```python
from build123d import *

# Parameters (mm, degrees)
SKETCH1_R                = 1.5
BOSS_EXTRUDE1_DEPTH      = 3.75
BOSS_EXTRUDE2_DEPTH      = 18
BOSS_EXTRUDE2_DEPTH_BACK = 7.5
CUT_EXTRUDE1_DEPTH       = 119.718371128
CUT_EXTRUDE1_DEPTH_BACK  = 3.5
SKETCH4_R                = 1.5
CHAMFER1_SIZE            = 2


with BuildPart() as part:
    # Sketch1 → Boss-Extrude1 (new, symmetric)
    with BuildSketch(Plane(origin=(0, 0, 0), x_dir=(1, 0, 0), z_dir=(0, 1, 0))):
        with BuildLine():
            Line((-14.064197212, 106.828183813), (-12.138935876, 92.204372108))
            ThreePointArc((-12.138935876, 92.204372108), (-8.327034738, 92.640714043), (-4.5, 92.914191088))
            Line((-4.5, 92.914191088), (-4.5, 90.60548378))
            Line((-4.5, 90.60548378), (-4.5, 89.092083998))
            Line((-4.5, 89.092083998), (-4.5, 87))
            ThreePointArc((-4.5, 87), (0, 82.5), (4.5, 87))
            Line((4.5, 87), (4.5, 89.092083998))
            Line((4.5, 89.092083998), (4.5, 90.60548378))
            Line((4.5, 90.60548378), (4.5, 92.914191088))
            ThreePointArc((4.5, 92.914191088), (8.327034738, 92.640714043), (12.138935876, 92.204372108))
            Line((12.138935876, 92.204372108), (14.064197212, 106.828183813))
            ThreePointArc((14.064197212, 106.828183813), (9.290945642, 107.337913445), (4.5, 107.638902983))
            Line((4.5, 107.638902983), (4.5, 109.907916002))
            Line((4.5, 109.907916002), (4.5, 112))
            ThreePointArc((4.5, 112), (0, 116.5), (-4.5, 112))
            Line((-4.5, 112), (-4.5, 109.907916002))
            Line((-4.5, 109.907916002), (-4.5, 107.638902983))
            ThreePointArc((-4.5, 107.638902983), (-9.290945642, 107.337913445), (-14.064197212, 106.828183813))
        make_face()
        with Locations(Location((0, 112, 0), (0, 0, 270))):
            Circle(SKETCH1_R, mode=Mode.SUBTRACT)
        with Locations(Location((0, 87, 0), (0, 0, 90))):
            Circle(SKETCH1_R, mode=Mode.SUBTRACT)
    extrude(amount=BOSS_EXTRUDE1_DEPTH, both=True)

    # Sketch3 → Boss-Extrude2 (add, two sides: drawn at the far end of the back side and taken through both)
    with BuildSketch(Plane(origin=(0, 3.75, 0), x_dir=(1, 0, 0), z_dir=(0, 1, 0)).offset(-BOSS_EXTRUDE2_DEPTH_BACK)):
        with BuildLine():
            Line((1.982080861, 94.766924481), (3.385996272, 105.430720736))
            ThreePointArc((3.385996272, 105.430720736), (2.964387866, 106.850395337), (1.636401853, 107.505897258))
            ThreePointArc((1.636401853, 107.505897258), (0, 107.524356631), (-1.636401853, 107.505897258))
            ThreePointArc((-1.636401853, 107.505897258), (-2.964387866, 106.850395337), (-3.385996272, 105.430720736))
            Line((-3.385996272, 105.430720736), (-1.982080861, 94.766924481))
            ThreePointArc((-1.982080861, 94.766924481), (-1.531449923, 93.718749438), (-0.551584549, 93.134281295))
            ThreePointArc((-0.551584549, 93.134281295), (-0.433742315, 93.139694116), (-0.315893802, 93.144968474))
            ThreePointArc((-0.315893802, 93.144968474), (1.206800808, 93.426480911), (1.982080861, 94.766924481))
        make_face()
    extrude(amount=BOSS_EXTRUDE2_DEPTH + BOSS_EXTRUDE2_DEPTH_BACK)

    # Sketch4 → Cut-Extrude1 (cut, two sides: drawn at the far end of the back side and taken through both)
    # profile 1 of 2: a face of its own
    with BuildSketch(Plane(origin=(0, 3.75, 0), x_dir=(1, 0, 0), z_dir=(0, 1, 0)).offset(-CUT_EXTRUDE1_DEPTH_BACK)):
        with BuildLine():
            Line((-4.5, 91.393652938), (-4.5, 87.032555921))
            ThreePointArc((-4.5, 87.032555921), (0, 82.41632562), (4.5, 87.032555921))
            Line((4.5, 87.032555921), (4.5, 91.393652938))
            Line((4.5, 91.393652938), (4.5, 92.914191088))
            Line((4.5, 92.914191088), (-4.5, 92.914191088))
            Line((-4.5, 92.914191088), (-4.5, 91.393652938))
        make_face()
        with Locations(Location((0, 87, 0), (0, 0, 90))):
            Circle(SKETCH4_R, mode=Mode.SUBTRACT)
    # profile 2 of 2: a face of its own
    with BuildSketch(Plane(origin=(0, 3.75, 0), x_dir=(1, 0, 0), z_dir=(0, 1, 0)).offset(-CUT_EXTRUDE1_DEPTH_BACK)):
        with BuildLine():
            Line((4.5, 107.638902983), (-4.5, 107.638902983))
            Line((-4.5, 107.638902983), (-4.5, 112))
            ThreePointArc((-4.5, 112), (0, 116.5), (4.5, 112))
            Line((4.5, 112), (4.5, 107.638902983))
        make_face()
        with Locations(Location((0, 112, 0), (0, 0, 270))):
            Circle(SKETCH4_R, mode=Mode.SUBTRACT)
    extrude(amount=CUT_EXTRUDE1_DEPTH + CUT_EXTRUDE1_DEPTH_BACK, mode=Mode.SUBTRACT)

    # Chamfer1
    chamfer1_edges = [part.edges().sort_by_distance(p)[0] for p in [
        (0, 0.25, -85.5),
        (0, 0.25, -113.5),
    ]]
    chamfer(chamfer1_edges, length=CHAMFER1_SIZE)

    # Chamfer2
    # the kernel refuses this chamfer: 1.5, 0.866025404 mm, written as the material it adds along each edge
    with BuildSketch(Plane(origin=(4.5, 0.25, -107.638902983), x_dir=(-1.576335496707441e-15, -0.057893862402670165, -0.9983227437537927), z_dir=(-1, 0, 0))) as chamfer2_piece_1:
        with BuildLine():
            Line((0.897530793, 0), (-0.119798729, -1.547621671))
            Line((-0.119798729, -1.547621671), (-0.149748412, -1.545884855))
            ThreePointArc((-0.149748412, -1.545884855), (-0.074874206, -0.772942428), (-0.029949682, 0.001736816))
            Line((-0.029949682, 0.001736816), (0.001736816, 0.029949682))
            ThreePointArc((0.001736816, 0.029949682), (0.448998086, 0.004012497), (0.899267609, 0.029949682))
            Line((0.899267609, 0.029949682), (0.897530793, 0))
        make_face()
    extrude(amount=9)
    with BuildSketch(Plane(origin=(4.5, 0.25, -92.914191088), x_dir=(0, 0.9998132206222078, -0.019326765612701434), z_dir=(-1, 0, 0))) as chamfer2_piece_2_section:
        with BuildLine():
            Line((1.552251453, 0), (-0.069269092, -0.894853797))
            Line((-0.069269092, -0.894853797), (-0.099263488, -0.894273994))
            ThreePointArc((-0.099263488, -0.894273994), (-0.038653033, -0.447349219), (-0.029994397, 0.000579803))
            Line((-0.029994397, 0.000579803), (0.000579803, 0.029994397))
            ThreePointArc((0.000579803, 0.029994397), (0.776415628, 0.014997198), (1.552831256, 0.029994397))
            Line((1.552831256, 0.029994397), (1.552251453, 0))
        make_face()
    chamfer2_piece_2 = extrude(amount=9, mode=Mode.PRIVATE)
    chamfer2_piece_2 = chamfer2_piece_2 & Plane(origin=(0, 0.749739916, -3.026761488), x_dir=(-0.13487706529406074, 0, -0.9908623402156638), z_dir=(0, 1, 0)) * Cylinder(90, 25, mode=Mode.PRIVATE)
    add(chamfer2_piece_2)


solid = part.part
```
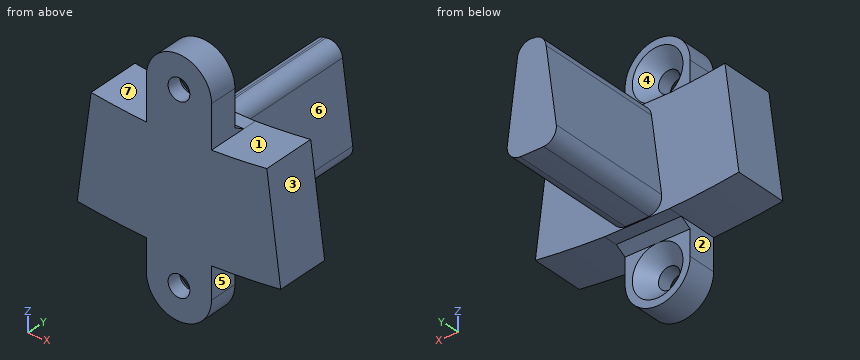
Build history of the part. All positions in model axes, mm. Face numbers are marked on the shaded views. A direction names the side the tool comes from. Give positions to 0.01 mm unless a question says otherwise; leave off trailing zeros. Loops run counter-clockwise (first coordinate to the right, second up) from the corner with the lowest first, then second, coordinate; pieces in that order, holes last. Notation, with made-up numbers: (78.25, -23.75) - (98.25, -23.75) arc R26 ccw to (98.25, -5.75) - close; hole circle Ø3 at (79.25, 74.25). An arc over 180 degrees is marked (long way). Use a Markdown table: item, result.
(1) Pull direction X, two halves, no side cores. Call the marked faces 1, 2 and 3: +X half, -X half, draft (parallel to the pull), parting line (faces both ways), or undercut.
Taken from the geometry:
| item | result |
|---|---|
| face 1 | undercut |
| face 2 | -X half |
| face 3 | +X half |
(2) Wall check: line 1 along X through (y, z) = (-3.25, -112); line 2 along Y through (x, z) = (-6, -101); line 3 along X through (y, z) = (11, -100). Give the ranges that are in metal, low to high.
Taken from the geometry:
| item | result |
|---|---|
| line 1 | -4.5 to -1.5, 1.5 to 4.5 |
| line 2 | -3.75 to 3.75 |
| line 3 | -2.67 to 2.67 |
(3) Band-saw the part on C-C (x = 9.25). Give the cut face in (y, z), and give its area (3 significant figures).
Taken from the geometry:
| item | result |
|---|---|
| outline | (-3.75, -107.34) - (3.75, -107.34) - (3.75, -92.55) - (-3.75, -92.55) - close |
| area | 111 mm2 |
(4) Band-saw the part on A-A (y = 12.5). Give the cut face in (x, z).
Taken from the geometry:
| item | result |
|---|---|
| outline | (-3.39, -105.43) arc R1.85 ccw to (-1.64, -107.51) arc R72.54 ccw to (1.64, -107.51) arc R1.85 ccw to (3.39, -105.43) - (1.98, -94.77) arc R1.85 ccw to (-0.32, -93.14) arc R100.4 cw to (-0.55, -93.13) arc R1.85 ccw to (-1.98, -94.77) - close |
(5) Which spindle directions (+Z, -Z, +X, -X, +Y, -Y) get a long thin tool onto all of the face, cutting with end or side? Do the marked faces 4, 5, 6 and 7. Say none if no direction does.
Taken from the geometry:
| item | result |
|---|---|
| face 4 | +Y |
| face 5 | -Z, +X, +Y, -Y |
| face 6 | +Z, +X, +Y |
| face 7 | +Z, +Y, -Y |
(6) Band-saw the part on B-B (z = -99). Give the cut face in (x, y), and give its area (3 significant figures).
Taken from the geometry:
| item | result |
|---|---|
| outline | (-13.03, -3.75) - (13.03, -3.75) - (13.03, 3.75) - (2.54, 3.75) - (2.54, 21.75) - (-2.54, 21.75) - (-2.54, 3.75) - (-13.03, 3.75) - close |
| area | 287 mm2 |
(7) Band-saw the part on D-D (y = 0.75). Give the cut face in (x, z), and give its area (3 significant figures).
Taken from the geometry:
| item | result |
|---|---|
| outline | (-14.06, -106.83) arc R110 ccw to (-4.5, -107.64) - (-4.5, -108.22) - (4.5, -108.22) - (4.5, -107.64) arc R110 ccw to (14.06, -106.83) - (12.14, -92.2) arc R90 cw to (4.5, -92.91) - (4.5, -92.34) - (-4.5, -92.34) - (-4.5, -92.91) arc R90 cw to (-12.14, -92.2) - close |
| area | 397 mm2 |
(8) Drop flat-ended pins along their axis: pin 1 Ø2 at (y, z) = (0, -110.5) entering from -X; pin 2 Ø8 at (y, z) = (16.5, -90.5) entering from -X; pin 3 Ø3 at (x, y) = (-2, 15.5) entering from +Z. Give the stop position or say it passes through.
Taken from the geometry:
| item | result |
|---|---|
| pin 1 | x = -4.5 |
| pin 2 | x = -1.94 |
| pin 3 | z = -93.13 |
